Check sheet for the drawn part. Datum: minimum x, y, z corner. Units: mm. Give positions to 0.01 mm unless a question says otherwise; leave off trailing zeros. Loops run counter-clockwise (first coordinate to the right, second up) from the corner with the lowest first, then second, coordinate; pieces in that order, holes last. Notation, with made-up numbers: (47.25, -3.5) - (99.25, -3.5) arc R10 cw to (99.25, 4.5) - close; hole circle Ø3 at (-4, 35). An arc over 180 degrees is marked (long way). One line per item, written item: value. Start each with the question number.
1. Sectioned sample at C-C (y = 30.5). Record the cut outline in (x, z), plus the area to 3 significant figures.
2. Scan lines: L1, parallel to X at y = 27, z = 6.25; L2, parallel to X at y = 17.5, z = 1.25 (1 decimal). Record each from-to range of solid material in increasing order. Write a range as [from, to].
3. Gauge pin test, flat ends, axial feed: pin 1 (2 mm diameter, centred on x = 8.5, y = 5.5, fed in from -Z) (1 decimal); pin 2 (2 mm diameter, centred on x = 7.5, y = 11, fed in from +Z); pin 3 (1 mm diameter, centred on x = 9, y = 3.5, fed in from +Z) (1 decimal). Record the tip position at first contact, or that the pin passes through.
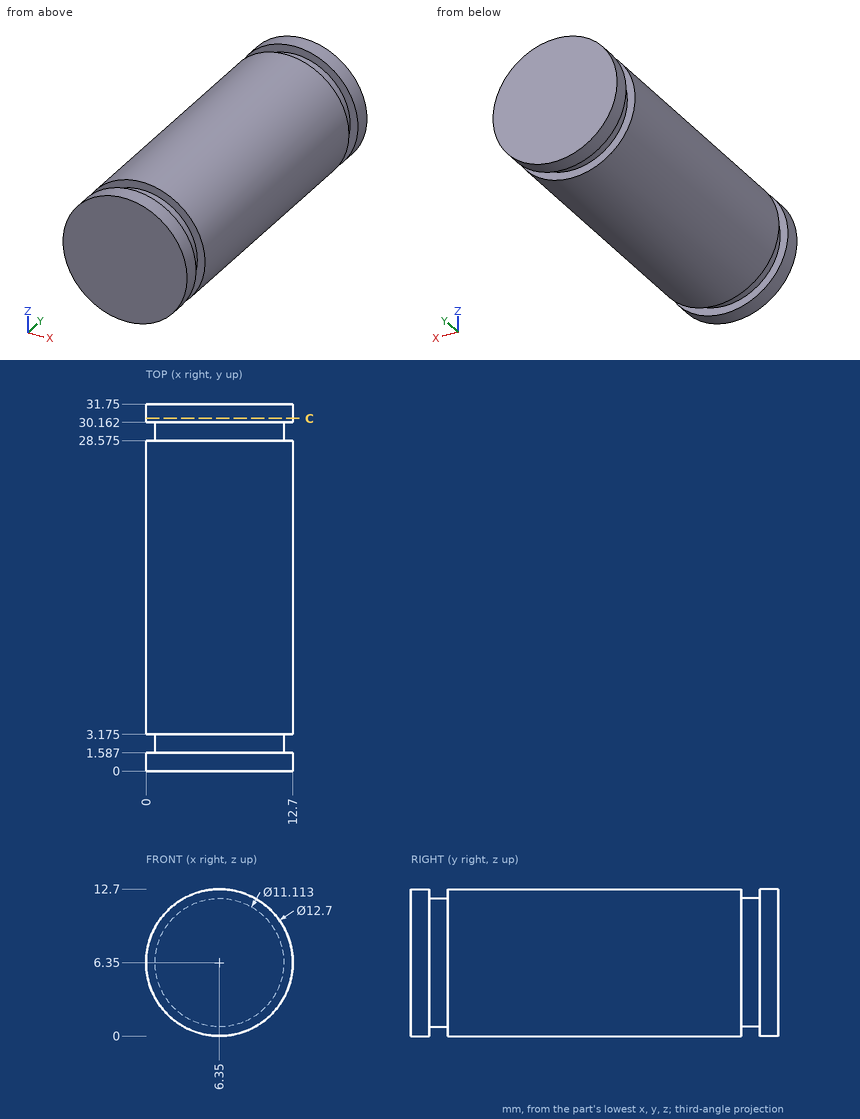
Results are:
1. outline: circle Ø12.7 at (6.35, 6.35)
1. area: 127 mm^2
2. L1: x = [0, 12.7]
2. L2: x = [2.6, 10.1]
3. pin 1: stops at z = 0.1
3. pin 2: stops at z = 12.7
3. pin 3: stops at z = 12.3
